Source: CAD feature listing. Evaluate the final solid. Frame: model axes, mm. A direction names the side the tool comes from. Coordinates: 2 decimals unless noted, no trailing zeros. Loops run counter-clockwise (first coordinate to the right, second up) from the corner with the lowest first, then second, coordinate; pieces in that order, holes last. Notation, with made-up numbers: M 55,5.5 L 70,5.5 A30 cw 70,32.5 Z; hole C 32.25,11.5 d11. An arc over 180 degrees is marked long. Write each question's results on one line, items separated by ' | '. Start each with the question number.
from build123d import *

# Parameters (mm, degrees)
SKETCH_1_R           = 38
EXTRUDE_1_DEPTH      = 150
SKETCH_2_R           = 10
EXTRUDE_2_DEPTH      = 36
SKETCH_3_OUTSIDE_W   = 148.554
SKETCH_3_OUTSIDE_H   = 148.554
SKETCH_3_OUTSIDE_W_2 = 16
SKETCH_3_OUTSIDE_H_2 = 16
CUT_EXTRUDE_1_DEPTH  = 38
HOLE_WIZARD_M10_1_D  = 8.5


with BuildPart() as part:
    # 草图1 → 凸台-拉伸1 (new, symmetric)
    with BuildSketch(Plane.XY):
        Circle(SKETCH_1_R)
    extrude(amount=EXTRUDE_1_DEPTH, both=True)

    # 草图2 → 凸台-拉伸2 (add)
    with BuildSketch(Plane.XY.offset(150)):
        Circle(SKETCH_2_R)
    extrude_2 = extrude(amount=EXTRUDE_2_DEPTH)

    # 草图3 outside → 切除-拉伸1 (cut)
    with BuildSketch(Plane.XY.offset(186)):
        Rectangle(SKETCH_3_OUTSIDE_W, SKETCH_3_OUTSIDE_H)
        Rectangle(SKETCH_3_OUTSIDE_W_2, SKETCH_3_OUTSIDE_H_2, mode=Mode.SUBTRACT)
    cut_extrude_1 = extrude(amount=-CUT_EXTRUDE_1_DEPTH, mode=Mode.SUBTRACT)

    # M10 螺纹孔1 (through all)
    with Locations(Plane.ZY.offset(8)):
        with Locations((172, 0)):
            hole_wizard_m10_1 = Hole(HOLE_WIZARD_M10_1_D / 2)

    # 镜向1: 凸台-拉伸2, 切除-拉伸1, M10 螺纹孔1 across plane
    add(extrude_2.mirror(Plane.XY))
    add(cut_extrude_1.mirror(Plane.XY), mode=Mode.SUBTRACT)
    add(hole_wizard_m10_1.mirror(Plane.XY), mode=Mode.SUBTRACT)


solid = part.part
Item 1: First-contact query: pin 1 Ø8 at (y, z) = (-28.5, 106.5) entering from -X; pin 2 Ø1 at (x, y) = (13, 21) entering from +Z; pin 3 Ø2 at (x, y) = (-7, 7.5) entering from -Z; pin 4 Ø13 at (x, z) = (3, 173.5) entering from -Y. Flat tips, straight axial feed; report the tip coordinate or a pass-through.
Item 2: Access query for faces 1 (the flat face through (0, -8, 167)), 2 (the flat face through (8, 0, -167)), 3 (the flat face through (0, -8, -167)). Directions: +Z, -Z, +X, -X, +Y, -Y. A direction counts if a zero-diameter tool reaches every point of the face in a straight line with its end or side. Return the directions, or none.
Item 3: Cut plane D-D (z = 53.5). Output: boundary loops of the cut face in (x, y).
Item 4: Mould query, pull axis Y, two halves, no side actions, for faces 4 (the flat face through (0, 8, 167)), 5 (the flat face through (-8, 0, 167)), 6 (the cylindrical face through (0.112, 0.187, -176.246)), 7 (the cylindrical face through (17.535, -33.713, 2.072)). Classes: +Y half, -Y half, draft (parallel to the pull), parting line (faces both ways), or undercut.
Item 5: Line query: probe 1 along Y at (x, z) = (-3, 172); probe 2 along Z at (x, y) = (3, -2.5); probe 3 along Z at (x, y) = (-20.5, 19). Output: solid intervals per line, ascending.
Item 6: Cut plane A-A (z = 172). Output: boundary loops of the cut face in (x, y).
Item 7: Cut plane B-B (y = 0). Output: boundary loops of the cut face in (x, z), then the cut area to 3 significant figures.
Item 8: Cut plane C-C (x = -21.5). Output: boundary loops of the cut face in (y, z).
Response values:
1) pin 1: stops at x = -29.05 | pin 2: stops at z = 148 | pin 3: stops at z = -186 | pin 4: stops at y = -8
2) face 1: +Z, +X, -X, -Y | face 2: -Z, +X, +Y, -Y | face 3: -Z, +X, -X, -Y
3) outline: C 0,0 d76
4) face 4: +Y half | face 5: draft | face 6: undercut | face 7: parting line
5) probe 1: y = -8 to -4.25, 4.25 to 8 | probe 2: z = -186 to -175.44, -168.56 to 168.56, 175.44 to 186 | probe 3: z = -148 to 148
6) outline: M -8,-6 A10 ccw -6,-8 L 6,-8 A10 ccw 8,-6 L 8,-4.25 L -8,-4.25 Z; M -8,4.25 L 8,4.25 L 8,6 A10 ccw 6,8 L -6,8 A10 ccw -8,6 Z
7) outline: M -38,-148 L -8,-148 L -8,-167.75 L 8,-167.75 L 8,-148 L 38,-148 L 38,148 L 8,148 L 8,167.75 L -8,167.75 L -8,148 L -38,148 Z; M -8,-186 L 8,-186 L 8,-176.25 L -8,-176.25 Z; M -8,176.25 L 8,176.25 L 8,186 L -8,186 Z | area: 23,400 mm2
8) outline: M -31.33,-148 L 31.33,-148 L 31.33,148 L -31.33,148 Z
